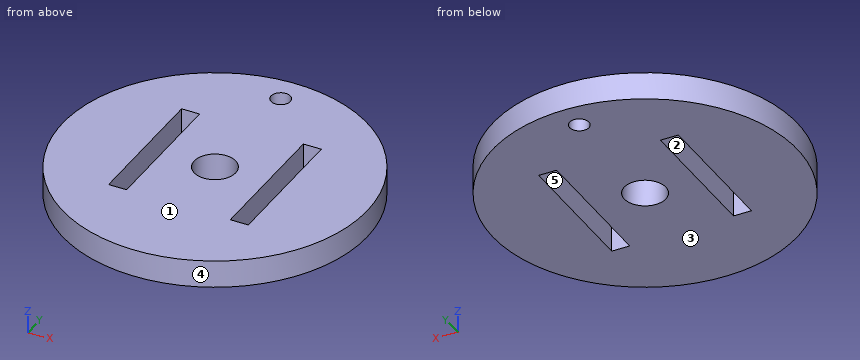
```python
from build123d import *

# Parameters (mm, degrees)
SKETCH1_R           = 11
SKETCH1_R_2         = 1.5
SKETCH1_R_3         = 0.7
SKETCH1_W           = 1.3
SKETCH1_H           = 10
BOSS_EXTRUDE1_DEPTH = 2


with BuildPart() as part:
    # Sketch1 → Boss-Extrude1 (new body)
    with BuildSketch(Plane.XY):
        Circle(SKETCH1_R)
        Circle(SKETCH1_R_2, mode=Mode.SUBTRACT)
        with Locations((0, 9)):
            Circle(SKETCH1_R_3, mode=Mode.SUBTRACT)
        with Locations((-4.4, 0)):
            Rectangle(SKETCH1_W, SKETCH1_H, mode=Mode.SUBTRACT)
        with Locations((4.4, 0)):
            Rectangle(SKETCH1_W, SKETCH1_H, mode=Mode.SUBTRACT)
    extrude(amount=BOSS_EXTRUDE1_DEPTH)


solid = part.part
```
Can you work these out from the model? Positions are in its coordinate system, mm. Face numbers are marked on the shaded views. A direction names the side the tool comes from. Round coordinates to 2 decimals unless told otherwise and drop trailing zeros. Loops run counter-clockwise (first coordinate to the right, second up) from the corner with the lowest first, then second, coordinate; pieces in that order, holes last.
Item 1: Which directions (+Z, -Z, +X, -X, +Y, -Y) give clear straight access to the entire face, cutting with the end or side of a thin tool? Please do the marked faces 1 and 2.
Item 2: Suppose I cut it at B-B, the plane x = 0. Write out the boundary of the cut face in (y, z).
Item 3: If we mould it in two halves opening along X, with no side actions, what happens to the marked faces 3, 4 and 5? For each: +X half, -X half, draft (parallel to the pull), parting line (faces both ways), or undercut.
Item 4: Suppose I cut it at C-C, the plane z = 1.3. Write out the boundary of the cut face in (x, y).
Item 5: Please list where these lines run through material, in increasing order: L1, parallel to Y at x = 0, z = 0.75; L2, parallel to Y at x = 4.5, z = 0.95; L3, parallel to X at y = 1, z = 1.3.
Item 6: Suppose I cut it at D-D, the plane y = 9. Write out the boundary of the cut face in (x, z), then the cut area to 3 significant figures.
Item 7: Suppose I cut it at A-A, the plane y = 0. Write out the boundary of the cut face in (x, z).
Item 8: Will these pins go through, and if not, where does the flat tip stop? pin 1 Ø1 at (x, z) = (2.5, 0.5) entering from -Y; pin 2 Ø0.6 at (y, z) = (2.5, 1) entering from +X; pin 3 Ø0.7 at (x, z) = (-4.5, 1) entering from +Y; pin 4 Ø1.1 at (x, y) = (0, 9) entering from +Z.
Reported:
1. face 1: +Z, +X, -X, +Y, -Y
1. face 2: +Z, -Z
2. outline: (-11, 0) - (-1.5, 0) - (-1.5, 2) - (-11, 2) - close; (1.5, 0) - (8.3, 0) - (8.3, 2) - (1.5, 2) - close; (9.7, 0) - (11, 0) - (11, 2) - (9.7, 2) - close
3. face 3: draft
3. face 4: parting line
3. face 5: undercut
4. outline: circle Ø22 at (0, 0); hole (-5.05, -5) - (-3.75, -5) - (-3.75, 5) - (-5.05, 5) - close; hole circle Ø3 at (0, 0); hole circle Ø1.4 at (0, 9); hole (3.75, -5) - (5.05, -5) - (5.05, 5) - (3.75, 5) - close
5. L1: y = -11 to -1.5, 1.5 to 8.3, 9.7 to 11
5. L2: y = -10.04 to -5, 5 to 10.04
5. L3: x = -10.95 to -5.05, -3.75 to -1.12, 1.12 to 3.75, 5.05 to 10.95
6. outline: (-6.32, 0) - (-0.7, 0) - (-0.7, 2) - (-6.32, 2) - close; (0.7, 0) - (6.32, 0) - (6.32, 2) - (0.7, 2) - close
6. area: 22.5 mm2
7. outline: (-11, 0) - (-5.05, 0) - (-5.05, 2) - (-11, 2) - close; (-3.75, 0) - (-1.5, 0) - (-1.5, 2) - (-3.75, 2) - close; (1.5, 0) - (3.75, 0) - (3.75, 2) - (1.5, 2) - close; (5.05, 0) - (11, 0) - (11, 2) - (5.05, 2) - close
8. pin 1: stops at y = -10.82
8. pin 2: stops at x = 10.78
8. pin 3: stops at y = 10.19
8. pin 4: passes through
